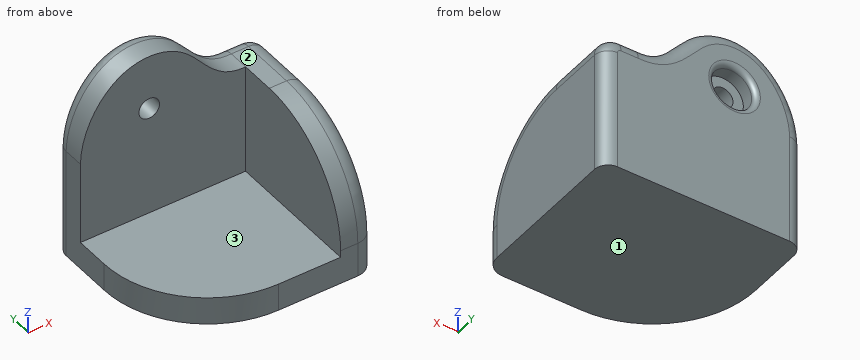
from build123d import *

# Parameters (mm, degrees)
F0_W     = 24
F0_H     = 4
F1_DEPTH = 25
F0_R     = 3
F0_R_2   = 1.5
F2_DEPTH = 5
F3_R     = 15
F4_R     = 2.5
F5_DEPTH = 2.5
F6_R     = 2
F7_R     = 0.75


with BuildPart() as f1:
    # F0 (on Front) → F1 (new body)
    with BuildSketch(Plane.XZ):
        with Locations((-12, 2)):
            Rectangle(F0_W, F0_H)
        Polygon((0, 20), (0, 4), (0, 0), (5, 0), (5, 20), align=None)
    extrude(amount=F1_DEPTH)

    # F0 (on Front) → F2 (join)
    with BuildSketch(Plane.XZ):
        with BuildLine():
            Line((-24, 16), (-24, 4))
            Line((-24, 4), (0, 4))
            Line((0, 4), (0, 20))
            add(Edge.make_bspline(
                [(-24, 16), (-23.9093121332, 20.5852864547), (-19.2329736628, 28.9244579006), (-7.5913408906, 27.8374196293), (-4.487070255, 19.7345465422), (0, 20)],
                knots=[0, 0, 0, 0, 0.3592153928, 0.6653798243, 1, 1, 1, 1], degree=3))
        make_face()
        with Locations((-14, 20)):
            Circle(F0_R, mode=Mode.SUBTRACT)
        with Locations((-12, 2)):
            Rectangle(F0_W, F0_H)
        Polygon((0, 20), (0, 4), (0, 0), (5, 0), (5, 20), align=None)
        with Locations((-14, 20)):
            Circle(F0_R)
        with Locations((-14, 20)):
            Circle(F0_R_2, mode=Mode.SUBTRACT)
    extrude(amount=F2_DEPTH)

    # F3
    f3_edges = [f1.edges().sort_by_distance(p)[0] for p in [
        (-24, -25, 2),
        (2.5, -25, 20),
    ]]
    fillet(f3_edges, radius=F3_R)

    # F4
    f4_edges = [f1.edges().sort_by_distance(p)[0] for p in [
        (5, -5, 20),
    ]]
    fillet(f4_edges, radius=F4_R)

    # F0 (on Front) → F5 (cut, symmetric)
    with BuildSketch(Plane.XZ):
        with Locations((-14, 20)):
            Circle(F0_R)
        with Locations((-14, 20)):
            Circle(F0_R_2, mode=Mode.SUBTRACT)
    extrude(amount=F5_DEPTH, both=True, mode=Mode.SUBTRACT)

    # F6
    f6_edges = [f1.edges().sort_by_distance(p)[0] for p in [
        (5, 0, 8.75),
        (4.267767, 0, 19.267767),
        (-24, 0, 8),
        (-14.21195, 0, 27.945974),
        (1.25, 0, 20),
    ]]
    fillet(f6_edges, radius=F6_R)

    # F7
    f7_edges = [f1.edges().sort_by_distance(p)[0] for p in [
        (-17, 0, 20),
    ]]
    fillet(f7_edges, radius=F7_R)


solid = f1.part
Model file for the job. Use its own axes, mm. Face numbers are marked on the shaded views. A direction names the side the tool comes from. Give positions to 0.01 mm unless a question says otherwise; leave off trailing zeros. Use CSV: the item, a comma, the result in double quotes.
1. 3-axis set-ups, long thin cutter, end or side, ignore diameter. For the marked faces 1, 2 and 3: which of +Z, -Z, +X, -X, +Y, -Y reach the whole face in a straight line?
Outcome:
face 1,"-Z, +X, -X, +Y, -Y"
face 2,"+Z, +X, +Y, -Y"
face 3,"+Z, -X, -Y"
2. Drill centre lines: line 1 along Z through (x, y) = (-14, -3.55); line 2 along X through (y, z) = (-6, 12.25); line 3 along Y through (x, z) = (-7.75, 4.5). Where is each one in solid material? Low to high. Write a range as from..to.
Outcome:
line 1,"0..18.5, 21.5..27.95"
line 2,"0..5"
line 3,"-5..0"
3. Drop flat-ended pins along their axis: pin 1 (5 mm diameter, centred on x = -14, z = 20, fed in from -Y); pin 2 (0.8 mm diameter, centred on x = 1.5, y = -5, fed in from +Z); pin 3 (1 mm diameter, centred on x = -17, y = -7, fed in from +Z); pin 4 (3 mm diameter, centred on x = 0.5, y = -13, fed in from -Z). Give the stop position or say it passes through.
Outcome:
pin 1,"y = -5"
pin 2,"z = 20"
pin 3,"z = 4"
pin 4,"z = 0"
